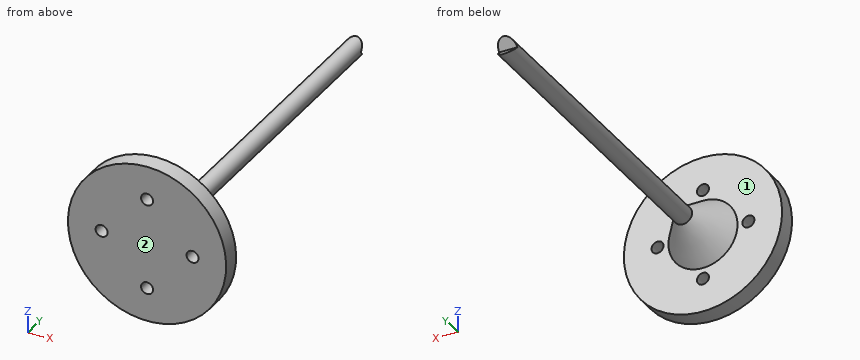
```python
from build123d import *

# Parameters (mm, degrees)
SKETCH1_R                = 43.5
BOSS_EXTRUDE4_DEPTH      = 10
HOLE_WIZARD_M6_2_D       = 6.6
CIRPATTERN1_COUNT        = 4
SKETCH20_R               = 5
BOSS_EXTRUDE6_DEPTH      = 200
CUT_EXTRUDE_1_DEPTH      = 10
CUT_EXTRUDE_1_DEPTH_BACK = 10
CHAMFER_1_SIZE           = 14
CHAMFER_1_SIZE2          = 19.994072094


with BuildPart() as part:
    # Sketch1 → Boss-Extrude4 (new body)
    with BuildSketch(Plane(origin=(0, 0, 0), x_dir=(1, 0, 0), z_dir=(0, 1, 0))):
        with Locations(Location((0, 0, 0), (0, 0, 270))):
            Circle(SKETCH1_R)
    extrude(amount=BOSS_EXTRUDE4_DEPTH)

    # Hole Wizard M6 _ _2 (through all)
    with Locations(Plane(origin=(0, 10, 0), x_dir=(1, 0, 0), z_dir=(0, 1, 0))):
        with Locations((0, -25)):
            hole_wizard_m6_2 = Hole(HOLE_WIZARD_M6_2_D / 2)

    # CirPattern1: Hole Wizard M6 _ _2 ×4 about axis
    cirpattern1_axis = Axis((0, 0, 0), (0, 1, 0))
    for i in range(1, CIRPATTERN1_COUNT):
        add(hole_wizard_m6_2.rotate(cirpattern1_axis, i * 360 / CIRPATTERN1_COUNT), mode=Mode.SUBTRACT)

    # Sketch20 → Boss-Extrude6 (add)
    with BuildSketch(Plane(origin=(0, 10, 0), x_dir=(1, 0, 0), z_dir=(0, 1, 0))):
        with Locations(Location((0, 0, 0), (0, 0, 270))):
            Circle(SKETCH20_R)
    extrude(amount=BOSS_EXTRUDE6_DEPTH)

    # Sketch 12 → Cut-Extrude 1 (cut, two sides: drawn at the far end of the back side and taken through both)
    with BuildSketch(Plane(origin=(0, 0, 0), x_dir=(0, 0, -1), z_dir=(1, 0, 0)).offset(-CUT_EXTRUDE_1_DEPTH_BACK)):
        Polygon((-5, 210), (5, 210), (0, 205), align=None)
    extrude(amount=CUT_EXTRUDE_1_DEPTH + CUT_EXTRUDE_1_DEPTH_BACK, mode=Mode.SUBTRACT)

    # Chamfer 1
    chamfer_1_edges = [part.edges().sort_by_distance(p)[0] for p in [
        (0, 10, -5),
    ]]
    chamfer_1_side = [part.faces().sort_by_distance(p)[0] for p in [
        (0, 10, -42.269634201),
    ]]
    chamfer(chamfer_1_edges, length=CHAMFER_1_SIZE, length2=CHAMFER_1_SIZE2, reference=chamfer_1_side[0])


solid = part.part
```
Verification items for the finished model (mm, model axes). Face numbers are marked on the shaded views. A direction names the side the tool comes from. Give positions to 0.01 mm unless a question says otherwise; leave off trailing zeros. Order: outer loops, then holes, each group sorted by start corner. A loop starts at its lowest first (then second) coordinate and runs counter-clockwise, first axis right, second up. Notation, with made-up numbers: (32, 13) - (84, 13) arc R20 cw to (84, 19) - close; hole circle Ø10 at (85, 70). An arc over 180 degrees is marked (long way). Answer as CSV lines item,"result". Start each with the question number.
Item 1: Access from +Z, -Z, +X, -X, +Y, -Y to the whole of each face (thin tool, end or side, straight path). Record for the marked faces 1 and 2.
Item 2: Material ranges on L1, parallel to X at y = 5.5, z = 0; L2, parallel to Y at x = -39, z = 10.5; L3, parallel to Z at x = 25, y = 7, recorded low to high.
Item 3: Gauge pin test, flat ends, axial feed: pin 1 (4 mm diameter, centred on x = 25, z = 0, fed in from -Y); pin 2 (10 mm diameter, centred on x = 7.5, y = 39.5, fed in from +Z); pin 3 (12 mm diameter, centred on y = 137.5, z = -3, fed in from -X). Record the tip position at first contact, or that the pin passes through.
Item 4: Section check C-C, the plane x = 25. Record the boundary of the cut face in (y, z).
Item 5: Section check A-A, the plane x = 0. Record the boundary of the cut face in (y, z), plus the area to 3 significant figures.
Item 6: Section check D-D, the plane y = 144. Record the boundary of the cut face in (x, z).
Item 7: Section check B-B, the plane z = -25. Record the boundary of the cut face in (x, y).
Filled in:
1,face 1,"+Y"
1,face 2,"+Z, -Z, +X, -X, -Y"
2,L1,"-43.5 to -28.3, -21.7 to 21.7, 28.3 to 43.5"
2,L2,"0 to 10"
2,L3,"-35.6 to -3.3, 3.3 to 35.6"
3,pin 1,"through"
3,pin 2,"z = 4.33"
3,pin 3,"x = -5"
4,outline,"(0, -35.6) - (10, -35.6) - (10, -3.3) - (0, -3.3) - close; (0, 3.3) - (10, 3.3) - (10, 35.6) - (0, 35.6) - close"
5,outline,"(0, -43.5) - (10, -43.5) - (10, -28.3) - (0, -28.3) - close; (0, -21.7) - (10, -21.7) - (10, -19) - (29.99, -5) - (210, -5) - (205, 0) - (210, 5) - (29.99, 5) - (10, 19) - (10, 21.7) - (0, 21.7) - close; (0, 28.3) - (10, 28.3) - (10, 43.5) - (0, 43.5) - close"
5,area,"2,990 mm^2"
6,outline,"circle Ø10 at (0, 0)"
7,outline,"(-35.6, 0) - (-3.3, 0) - (-3.3, 10) - (-35.6, 10) - close; (3.3, 0) - (35.6, 0) - (35.6, 10) - (3.3, 10) - close"
